```python
from build123d import *

# Parameters (mm, degrees)
F0_W         = 150
F0_H         = 150
F1_DEPTH     = 3
F2_W         = 89.5
F2_H         = 60.5
F2_W_2       = 85.5
F2_H_2       = 56.5
F3_DEPTH     = 3
F4_W         = 12
F4_H         = 2
F4_W_2       = 2
F4_H_2       = 15
F5_DEPTH     = 3
F6_R         = 5
F7_W         = 89.5
F7_H         = 59.5
F7_W_2       = 85.5
F7_H_2       = 55.5
F8_DEPTH     = 3
F9_R         = 3.6271227465
F9_R_2       = 2.5
F9_R_3       = 3.5
F10_DEPTH    = 70
F12_DEPTH    = 3
F13_R        = 2.5
F13_R_2      = 28.6222607242
F13_R_3      = 34.4815327899
F13_R_4      = 36.1444775831
F14_DEPTH    = 25
F16_DEPTH    = 25
F17_T1_DEPTH = 3
F18_R        = 1.375
F19_DEPTH    = 25
F20_W        = 2.75
F20_H        = 2
F21_DEPTH    = 25
F23_R        = 1.375
F24_DEPTH    = 25
F26_DEPTH    = 25


# Not quite as in the source:
# - a fillet or chamfer that OpenCascade refuses, or shapes differently, is made with other operations: its cross-section is extruded or revolved along the edge and cut away or added


with BuildPart() as f1:
    # F0 (on Top) → F1 (new body)
    with BuildSketch(Plane.XY):
        Rectangle(F0_W, F0_H)
    extrude(amount=F1_DEPTH)

    # F2 (on face) → F3 (join)
    with BuildSketch(Plane.XY.offset(3)):
        with Locations((20.25, 33.25)):
            Rectangle(F2_W, F2_H)
        with Locations((20.25, 33.25)):
            Rectangle(F2_W_2, F2_H_2, mode=Mode.SUBTRACT)
    extrude(amount=F3_DEPTH)

    # F4 (on face) → F5 (cut)
    with BuildSketch(Plane.XY.offset(6)):
        with Locations((52.15, 62.5)):
            Rectangle(F4_W, F4_H)
        with Locations((64, 33.25)):
            Rectangle(F4_W_2, F4_H_2)
    extrude(amount=-F5_DEPTH, mode=Mode.SUBTRACT)

    # F6
    f6_edges = [f1.edges().sort_by_distance(p)[0] for p in [
        (-75, 75, 1.5),
        (75, 75, 1.5),
        (75, -75, 1.5),
        (-75, -75, 1.5),
    ]]
    fillet(f6_edges, radius=F6_R)

    # F7 (on face) → F8 (join)
    with BuildSketch(Plane.XY.offset(3)):
        with Locations((20.25, -32.75)):
            Rectangle(F7_W, F7_H)
        with Locations((20.25, -32.75)):
            Rectangle(F7_W_2, F7_H_2, mode=Mode.SUBTRACT)
    extrude(amount=F8_DEPTH)

    # F9 (on face) → F10 (join)
    with BuildSketch(Plane.XY.offset(3)):
        with Locations((68.8578643763, 60.8578643763)):
            Circle(F9_R)
        with Locations((68.8578643763, 60.8578643763)):
            Circle(F9_R_2, mode=Mode.SUBTRACT)
        with Locations((68.8578643763, -60.8578643763)):
            Circle(F9_R)
        with Locations((68.8578643763, -60.8578643763)):
            Circle(F9_R_2, mode=Mode.SUBTRACT)
        with Locations((-52.8578643763, 60.8578643763)):
            Circle(F9_R_3)
        with Locations((-52.8578643763, 60.8578643763)):
            Circle(F9_R_2, mode=Mode.SUBTRACT)
        with Locations((-52.8578643763, -60.8578643763)):
            Circle(F9_R_3)
        with Locations((-52.8578643763, -60.8578643763)):
            Circle(F9_R_2, mode=Mode.SUBTRACT)
    extrude(amount=F10_DEPTH)

    # F11 (on face) → F12 (join)
    with BuildSketch(Plane.XY.offset(3)):
        Polygon((-1.4142135624, 2.1213203436), (-2.1213203436, 1.4142135624), (-0.7071067812, 0), (-2.1213203436, -1.4142135624), (-1.4142135624, -2.1213203436), (0, -0.7071067812), (1.4142135624, -2.1213203436), (2.1213203436, -1.4142135624), (0.7071067812, 0), (2.1213203436, 1.4142135624), (1.4142135624, 2.1213203436), (0, 0.7071067812), align=None)
    extrude(amount=F12_DEPTH)

    # F13 (on face) → F14 (cut)
    with BuildSketch(Plane.XY.offset(3)):
        with Locations((-52.8578643763, 60.8578643763)):
            Circle(F13_R)
        with Locations((662.2217056946, 102.264947845)):
            Circle(F13_R_2)
        with Locations((693.5295645663, -597.344861617)):
            Circle(F13_R_3)
        with Locations((-44.6129470708, -626.2444101651)):
            Circle(F13_R_4)
        with Locations((68.8578643763, 60.8578643763)):
            Circle(F13_R)
        with Locations((68.8578643763, -60.8578643763)):
            Circle(F13_R)
        with Locations((-52.8578643763, -60.8578643763)):
            Circle(F13_R)
    extrude(amount=-F14_DEPTH, mode=Mode.SUBTRACT)

    # F15 (on face) → F16 (cut)
    with BuildSketch(Plane.XY.offset(3)):
        Polygon((-24.5, 19.5), (-75, 70), (-75, -70), (-24.5, -19.5), align=None)
    extrude(amount=-F16_DEPTH, mode=Mode.SUBTRACT)

    # F17: fillet of radius 5 on 4 edges, made by hand

    # F17_s2 → F17_t1 (join)
    with BuildSketch(Plane.XY):
        with BuildLine():
            ThreePointArc((-24.5, 17.4289321881), (-24.8806023374, 19.34234935), (-25.9644660941, 20.9644660941))
            Line((-25.9644660941, 20.9644660941), (-24.5, 19.5))
            Line((-24.5, 19.5), (-24.5, 17.4289321881))
        make_face()
        with BuildLine():
            ThreePointArc((-25.9644660941, -20.9644660941), (-24.8806023374, -19.34234935), (-24.5, -17.4289321881))
            Line((-24.5, -17.4289321881), (-24.5, -19.5))
            Line((-24.5, -19.5), (-25.9644660941, -20.9644660941))
        make_face()
    extrude(amount=F17_T1_DEPTH)

    # F18 (on face) → F19 (cut)
    with BuildSketch(Plane.XY.offset(6)):
        with Locations((-18.5, 57.5)):
            Circle(F18_R)
        with Locations((39.5, 58)):
            Circle(F18_R)
        with Locations((-19, 8.5)):
            Circle(F18_R)
        with Locations((39, 8.5)):
            Circle(F18_R)
    extrude(amount=-F19_DEPTH, mode=Mode.SUBTRACT)

    # F20 (on face) → F21 (cut)
    with BuildSketch(Plane.XY.offset(6)):
        with Locations((-18.525, 62.5)):
            Rectangle(F20_W, F20_H)
        with Locations((39.425, 62.5)):
            Rectangle(F20_W, F20_H)
        with Locations((39.025, 4)):
            Rectangle(F20_W, F20_H)
        with Locations((-19.025, 4)):
            Rectangle(F20_W, F20_H)
    extrude(amount=-F21_DEPTH, mode=Mode.SUBTRACT)

    # F23 (on face) → F24 (cut)
    with BuildSketch(Plane.XY.offset(3)):
        with Locations((-4.75, 0)):
            Circle(F23_R)
        with Locations((20.25, 0)):
            Circle(F23_R)
        with Locations((45.25, 0)):
            Circle(F23_R)
        with Locations((45.25, -65.5)):
            Circle(F23_R)
        with Locations((20.25, -65.5)):
            Circle(F23_R)
        with Locations((-4.75, -65.5)):
            Circle(F23_R)
    extrude(amount=-F24_DEPTH, mode=Mode.SUBTRACT)

    # F25 (on face) → F26 (cut)
    with BuildSketch(Plane.XY.offset(6)):
        with BuildLine():
            Line((48.8800137441, 16.2271423447), (26.3292788436, 45.2489576949))
            ThreePointArc((26.3292788436, 45.2489576949), (24.1013697846, 45.9137135619), (22.75, 44.0218153502))
            Line((22.75, 44.0218153502), (22.75, 15))
            ThreePointArc((22.75, 15), (23.3357864376, 13.5857864376), (24.75, 13))
            Line((24.75, 13), (47.3007349005, 13))
            ThreePointArc((47.3007349005, 13), (49.0971597792, 14.120876769), (48.8800137441, 16.2271423447))
        make_face()
        with BuildLine():
            Line((28.7575768219, 50.2728576553), (51.4207211564, 21.1063762509))
            ThreePointArc((51.4207211564, 21.1063762509), (53.6486302154, 20.4416203838), (55, 22.3335185956))
            Line((55, 22.3335185956), (55, 51.5))
            ThreePointArc((55, 51.5), (54.4142135624, 52.9142135624), (53, 53.5))
            Line((53, 53.5), (30.3368556655, 53.5))
            ThreePointArc((30.3368556655, 53.5), (28.5404307868, 52.379123231), (28.7575768219, 50.2728576553))
        make_face()
        with BuildLine():
            ThreePointArc((-12.5, 53.5), (-13.9142135624, 52.9142135624), (-14.5, 51.5))
            Line((-14.5, 51.5), (-14.5, 22.3335185956))
            ThreePointArc((-14.5, 22.3335185956), (-13.1486302154, 20.4416203838), (-10.9207211564, 21.1063762509))
            Line((-10.9207211564, 21.1063762509), (11.7424231781, 50.2728576553))
            ThreePointArc((11.7424231781, 50.2728576553), (11.9595692132, 52.379123231), (10.1631443345, 53.5))
            Line((10.1631443345, 53.5), (-12.5, 53.5))
        make_face()
        with BuildLine():
            Line((17.75, 15), (17.75, 44.0218153502))
            ThreePointArc((17.75, 44.0218153502), (16.3986302154, 45.9137135619), (14.1707211564, 45.2489576949))
            Line((14.1707211564, 45.2489576949), (-8.3800137441, 16.2271423447))
            ThreePointArc((-8.3800137441, 16.2271423447), (-8.5971597792, 14.120876769), (-6.8007349005, 13))
            Line((-6.8007349005, 13), (15.75, 13))
            ThreePointArc((15.75, 13), (17.1642135624, 13.5857864376), (17.75, 15))
        make_face()
        with BuildLine():
            Line((-14.5, -22.3335185956), (-14.5, -51.5))
            ThreePointArc((-14.5, -51.5), (-13.9142135624, -52.9142135624), (-12.5, -53.5))
            Line((-12.5, -53.5), (10.1631443345, -53.5))
            ThreePointArc((10.1631443345, -53.5), (11.9595692132, -52.379123231), (11.7424231781, -50.2728576553))
            Line((11.7424231781, -50.2728576553), (-10.9207211564, -21.1063762509))
            ThreePointArc((-10.9207211564, -21.1063762509), (-13.1486302154, -20.4416203838), (-14.5, -22.3335185956))
        make_face()
        with BuildLine():
            ThreePointArc((24.75, -13), (23.3357864376, -13.5857864376), (22.75, -15))
            Line((22.75, -15), (22.75, -44.0218153502))
            ThreePointArc((22.75, -44.0218153502), (24.1013697846, -45.9137135619), (26.3292788436, -45.2489576949))
            Line((26.3292788436, -45.2489576949), (48.8800137441, -16.2271423447))
            ThreePointArc((48.8800137441, -16.2271423447), (49.0971597792, -14.120876769), (47.3007349005, -13))
            Line((47.3007349005, -13), (24.75, -13))
        make_face()
        with BuildLine():
            ThreePointArc((53, -53.5), (54.4142135624, -52.9142135624), (55, -51.5))
            Line((55, -51.5), (55, -22.3335185956))
            ThreePointArc((55, -22.3335185956), (53.6486302154, -20.4416203838), (51.4207211564, -21.1063762509))
            Line((51.4207211564, -21.1063762509), (28.7575768219, -50.2728576553))
            ThreePointArc((28.7575768219, -50.2728576553), (28.5404307868, -52.379123231), (30.3368556655, -53.5))
            Line((30.3368556655, -53.5), (53, -53.5))
        make_face()
        with BuildLine():
            Line((17.75, -44.0218153502), (17.75, -15))
            ThreePointArc((17.75, -15), (17.1642135624, -13.5857864376), (15.75, -13))
            Line((15.75, -13), (-6.8007349005, -13))
            ThreePointArc((-6.8007349005, -13), (-8.5971597792, -14.120876769), (-8.3800137441, -16.2271423447))
            Line((-8.3800137441, -16.2271423447), (14.1707211564, -45.2489576949))
            ThreePointArc((14.1707211564, -45.2489576949), (16.3986302154, -45.9137135619), (17.75, -44.0218153502))
        make_face()
    extrude(amount=-F26_DEPTH, mode=Mode.SUBTRACT)


solid = f1.part
```
Check sheet for the modelled part. Datum: model origin and axes. Units: mm. A direction names the side the tool comes from. Give positions to 0.01 mm unless a question says otherwise; leave off trailing zeros. Write each loop counter-clockwise with the first axis right and the second up, starting at its lowest first coordinate (ties: lowest second). Pieces come first, ordered by that corner, then holes. Notation, with made-up numbers: (32.25, 78) - (80.25, 78) arc R19 ccw to (80.25, 87) - close; hole circle Ø7 at (73, -1.5). An arc over 180 degrees is marked (long way). Answer as a JSON object with one key per item and string values. Group by question number.
1) Access from +Z, -Z, +X, -X, +Y, -Y to the whole of each face (thin tool, end or side, straight path). Record for faces 4 (the face through (20, -32, 3)), 5 (the face through (-51, -46, 2)), 6 (the face through (40.248, -35.485, 1.521)), 7 (the face through (64, 55, 6)).
2) Thickness scan on probe 1 along Y at (x, z) = (-51, 6); probe 2 along X at (y, z) = (17.5, 5); probe 3 along X at (y, z) = (-65.5, 0.6) (3 decimals). Record the ranges inside material, lowest first. Write a range as from..to.
3) Depth check by flat-ended pin: P1, Ø2.5, axis at y = 54.5, z = 5, coming from the -X side; P2, Ø1.6, axis at x = 63.5, z = 4, coming from the -Y side; P3, Ø12, axis at x = 28, y = 13, coming from the +Z side. Enter the tip coordinate at first touch or a pass-through.
4) Release check for a two-part mould opening along X. For faces 1 (the face through (66, -62, 73)), 2 (the face through (2.737, -30.535, 1.521)), 3 (the face through (73, 74, 2)) record: pulls with the +X half, pulls with the -X half, needs draft (parallel to the pull), parting line crosses it, or undercut.
5) Sectioned sample at A-A (z = 16). Record the cut outline in (x, y), then the cut area to 3 significant figures.
Geometry results:
{
 "1": {"face 4": "+Z", "face 5": "+Z, -Z, -X", "face 6": "+Z, -Z", "face 7": "+Z, +Y, -Y"},
 "2": {"probe 1": "y = -63.82..-62.53, -59.19..-57.89, 57.89..59.19, 62.53..63.82", "probe 2": "x = -24.5..-22.5, 63..65", "probe 3": "x = -70.5..-6.125, -3.375..18.875, 21.625..43.875, 46.625..75"},
 "3": {"P1": "stops at x = -24.5", "P2": "stops at y = -62.5", "P3": "stops at z = 3"},
 "4": {"face 1": "needs draft", "face 2": "undercut", "face 3": "pulls with the +X half"},
 "5": {"outline": "circle Ø7 at (-52.86, -60.86); circle Ø7 at (-52.86, 60.86); circle Ø7.25 at (68.86, -60.86); circle Ø7.25 at (68.86, 60.86); hole circle Ø5 at (-52.86, -60.86); hole circle Ø5 at (-52.86, 60.86); hole circle Ø5 at (68.86, -60.86); hole circle Ø5 at (68.86, 60.86)", "area": "81.1 mm^2"}
}
